CAD build for the part. Positions are in the model's coordinates, mm. Coordinates: 2 decimals unless noted, no trailing zeros. Loops run counter-clockwise (first coordinate to the right, second up) from the corner with the lowest first, then second, coordinate; pieces in that order, holes last. Notation, with made-up numbers: (76, -14.5) - (120, -14.5) arc R30 ccw to (120, 11.5) - close; hole circle Ø3 at (17, 50.5). An arc over 180 degrees is marked (long way). Put each result on its own line as item: value.
```python
from build123d import *

# Parameters (mm, degrees)
SKETCH1_W           = 195
SKETCH1_H           = 120.54
SKETCH1_R           = 1.75
BOSS_EXTRUDE1_DEPTH = 3
FILLET1_R           = 1
SKETCH3_W           = 5
SKETCH3_H           = 100
CUT_EXTRUDE1_DEPTH  = 230.268165256


with BuildPart() as part:
    # Sketch1 → Boss-Extrude1 (new body)
    with BuildSketch(Plane.XY):
        with Locations((97.5, 60.27)):
            Rectangle(SKETCH1_W, SKETCH1_H)
        with Locations((4, 116.54)):
            Circle(SKETCH1_R, mode=Mode.SUBTRACT)
        with Locations((191, 116.54)):
            Circle(SKETCH1_R, mode=Mode.SUBTRACT)
        with Locations((4, 4)):
            Circle(SKETCH1_R, mode=Mode.SUBTRACT)
        with Locations((191, 4)):
            Circle(SKETCH1_R, mode=Mode.SUBTRACT)
    extrude(amount=BOSS_EXTRUDE1_DEPTH)

    # Fillet1
    fillet1_edges = [part.edges().sort_by_distance(p)[0] for p in [
        (195, 60.27, 3),
        (97.5, 120.54, 3),
        (0, 60.27, 3),
        (97.5, 120.54, 0),
        (195, 60.27, 0),
        (97.5, 0, 0),
        (0, 60.27, 0),
        (0, 120.54, 1.5),
        (195, 120.54, 1.5),
        (195, 0, 1.5),
        (0, 0, 1.5),
        (97.5, 0, 3),
    ]]
    fillet(fillet1_edges, radius=FILLET1_R)

    # Sketch3 → Cut-Extrude1 (cut, through all)
    with BuildSketch(Plane.XY.offset(3)):
        with Locations((27.5, 60.27)):
            Rectangle(SKETCH3_W, SKETCH3_H)
        with Locations((17.5, 60.27)):
            Rectangle(SKETCH3_W, SKETCH3_H)
        with Locations((37.5, 60.27)):
            Rectangle(SKETCH3_W, SKETCH3_H)
        with Locations((47.5, 60.27)):
            Rectangle(SKETCH3_W, SKETCH3_H)
        with Locations((57.5, 60.27)):
            Rectangle(SKETCH3_W, SKETCH3_H)
        with Locations((67.5, 60.27)):
            Rectangle(SKETCH3_W, SKETCH3_H)
        with Locations((77.5, 60.27)):
            Rectangle(SKETCH3_W, SKETCH3_H)
        with Locations((87.5, 60.27)):
            Rectangle(SKETCH3_W, SKETCH3_H)
        with Locations((97.5, 60.27)):
            Rectangle(SKETCH3_W, SKETCH3_H)
        with Locations((107.5, 60.27)):
            Rectangle(SKETCH3_W, SKETCH3_H)
        with Locations((117.5, 60.27)):
            Rectangle(SKETCH3_W, SKETCH3_H)
        with Locations((127.5, 60.27)):
            Rectangle(SKETCH3_W, SKETCH3_H)
        with Locations((137.5, 60.27)):
            Rectangle(SKETCH3_W, SKETCH3_H)
        with Locations((147.5, 60.27)):
            Rectangle(SKETCH3_W, SKETCH3_H)
        with Locations((157.5, 60.27)):
            Rectangle(SKETCH3_W, SKETCH3_H)
        with Locations((167.5, 60.27)):
            Rectangle(SKETCH3_W, SKETCH3_H)
        with Locations((177.5, 60.27)):
            Rectangle(SKETCH3_W, SKETCH3_H)
    extrude(amount=-CUT_EXTRUDE1_DEPTH, mode=Mode.SUBTRACT)


solid = part.part
```
Q1. Mould opens along Y. For faces 1 (the cylindrical face through (3.62, 114.83, 1.48)), 2 (the flat face through (74.7, 61.1, 3)) say: +Y half, -Y half, draft (parallel to the pull), parting line (faces both ways), or undercut.
Determined:
face 1: undercut
face 2: draft
Q2. Slice it at B-B, the plane y = 33. State how many separate pieces and enclosed holes the cut face has, then the cut area to 3 significant figures.
Determined:
separate pieces: 18
enclosed holes: 0
area: 329 mm2
Q3. Wall check: L1, parallel to X at y = 116.54, z = 2.1; L2, parallel to Y at x = 128.5, z = 1.95; L3, parallel to Y at x = 191, z = 1.35. Give the ranges that are in metal, low to high. Write a range as from..to.
Determined:
L1: 0.01..2.25, 5.75..189.25, 192.75..194.99
L2: 0..10.27, 110.27..120.54
L3: 0..2.25, 5.75..114.79, 118.29..120.54
Q4. Slice it at A-A, the plane x = 147. Give the cut face in (y, z), then the cut area to 3 significant figures.
Determined:
outline: (0, 1) arc R1 ccw to (1, 0) - (10.27, 0) - (10.27, 3) - (1, 3) arc R1 ccw to (0, 2) - close; (110.27, 0) - (119.54, 0) arc R1 ccw to (120.54, 1) - (120.54, 2) arc R1 ccw to (119.54, 3) - (110.27, 3) - close
area: 60.8 mm2
